Geometry check sheet. Reference: the model listing, model coordinates, mm. Coordinates: 2 decimals unless noted, no trailing zeros. Write each loop counter-clockwise with the first axis right and the second up, starting at its lowest first coordinate (ties: lowest second). Pieces come first, ordered by that corner, then holes. Notation, with made-up numbers: (-18.5, 43.25) -> (-9.5, 43.25) arc R29 ccw to (-9.5, 77.25) -> close; hole circle Ø11 at (41, -29). An arc over 180 degrees is marked (long way). Answer as CSV lines item,"result".
```python
from build123d import *

# Parameters (mm, degrees)
F1_DEPTH = 3
F2_DEPTH = 25
F3_R     = 7
F4_R     = 100
F5_R     = 7
F6_R     = 3


# Not quite as in the source:
# - a feature names something its author has since deleted; it is built from what else it names


with BuildPart() as f1:
    # F0 (on Front) → F1 (new body)
    with BuildSketch(Plane.XZ):
        with BuildLine():
            Line((-28.5062876117, 71.7030383349), (-23.3711215756, 71.5975238881))
            ThreePointArc((-23.3711215756, 71.5975238881), (-24.6315082315, 75.5227380174), (-26.6928125912, 79.0930187933))
            ThreePointArc((-26.6928125912, 79.0930187933), (-46.4685424733, 86.625019162), (-61.3664115867, 71.5962461648))
            Line((-61.3664115867, 71.5962461648), (-56.3664115867, 71.5913571682))
            ThreePointArc((-56.3664115867, 71.5913571682), (-42.4756351566, 81.447422187), (-28.5062876117, 71.7030383349))
        make_face()
        with BuildLine():
            ThreePointArc((-61.3664115867, 71.5962461648), (-42.3681277411, 52.5998806027), (-23.3711215756, 71.5975238881))
            Line((-23.3711215756, 71.5975238881), (-28.5062876117, 71.7030383349))
            ThreePointArc((-28.5062876117, 71.7030383349), (-35.0280474509, 67.9936357913), (-42.4162418185, 66.6868830915))
            ThreePointArc((-42.4162418185, 66.6868830915), (-49.8149115034, 67.9342855664), (-56.3664115867, 71.5913571682))
            Line((-56.3664115867, 71.5913571682), (-61.3664115867, 71.5962461648))
        make_face()
        with BuildLine():
            ThreePointArc((-42.4162418185, 66.6868830915), (-35.0280474509, 67.9936357913), (-28.5062876117, 71.7030383349))
            ThreePointArc((-28.5062876117, 71.7030383349), (-42.4756351566, 81.447422187), (-56.3664115867, 71.5913571682))
            ThreePointArc((-56.3664115867, 71.5913571682), (-49.8149115034, 67.9342855664), (-42.4162418185, 66.6868830915))
        make_face()
        with BuildLine():
            Line((-20.8711215756, 71.5975236603), (-23.3711215756, 71.5975238881))
            ThreePointArc((-23.3711215756, 71.5975238881), (-42.3681277411, 52.5998806027), (-61.3664115867, 71.5962461648))
            Line((-61.3664115867, 71.5962461648), (-63.866411581, 71.5960777947))
            ThreePointArc((-63.866411581, 71.5960777947), (-63.6941147241, 68.8812286525), (-63.1803487139, 66.2098738354))
            ThreePointArc((-63.1803487139, 66.2098738354), (-48.9397473345, 51.1287456375), (-28.5819229469, 55.1029300277))
            ThreePointArc((-28.5819229469, 55.1029300277), (-22.8939959961, 62.4935676044), (-20.8711215756, 71.5975236602))
        make_face()
        with BuildLine():
            ThreePointArc((-26.6928125912, 79.0930187933), (-24.6315082315, 75.5227380174), (-23.3711215756, 71.5975238881))
            Line((-23.3711215756, 71.5975238881), (-20.8711215756, 71.5975236603))
            ThreePointArc((-20.8711215756, 71.5975236602), (-22.8939959961, 62.4935676044), (-28.5819229469, 55.1029300277))
            ThreePointArc((-28.5819229469, 55.1029300277), (-33.5715090435, 45.0303149316), (-38.6320985636, 34.9931849634))
            ThreePointArc((-38.6320985636, 34.9931849634), (-28.2353261857, 40.6242290748), (-18.8527258187, 47.819251244))
            ThreePointArc((-18.8527258187, 47.819251244), (-11.5073907557, 58.7139707043), (-8.9261215756, 71.5975225718))
            Line((-8.9261215756, 71.5975225718), (-11.6744206899, 71.5975225718))
            Line((-11.6744206899, 71.5975225718), (-11.6744206899, 74.0203762137))
            ThreePointArc((-11.6744206899, 74.0203762137), (-14.431706638, 81.8781100982), (-19.1607128583, 88.7325325952))
            ThreePointArc((-19.1607128583, 88.7325325952), (-48.5320541227, 98.3962580044), (-71.9061774941, 78.1548738354))
            Line((-71.9061774941, 78.1548738354), (-107.2845857728, 78.1548738354))
            Line((-107.2845857728, 78.1548738354), (-119.2295857724, 78.1548738354))
            Line((-119.2295857724, 78.1548738354), (-119.2295857724, 66.2098738355))
            Line((-119.2295857724, 66.2098738355), (-119.2295857724, 47.819251244))
            ThreePointArc((-119.2295857724, 47.819251244), (-113.3445755267, 44.456364285), (-107.2845857724, 41.4201036786))
            Line((-107.2845857724, 41.4201036786), (-107.2845857724, 66.2098738354))
            Line((-107.2845857724, 66.2098738354), (-68.5864427672, 66.2098738354))
            Line((-68.5864427672, 66.2098738354), (-63.1803487138, 66.2098738354))
            ThreePointArc((-63.1803487139, 66.2098738354), (-63.6941147241, 68.8812286525), (-63.866411581, 71.5960777947))
            Line((-63.866411581, 71.5960777947), (-61.3664115867, 71.5962461648))
            ThreePointArc((-61.3664115867, 71.5962461648), (-46.4685424733, 86.625019162), (-26.6928125912, 79.0930187933))
        make_face()
        with BuildLine():
            Line((-11.6744206899, 71.5975225718), (-8.9261215756, 71.5975225718))
            ThreePointArc((-8.9261215756, 71.5975225718), (-13.1797411051, 80.6808937542), (-19.1607128583, 88.7325325952))
            ThreePointArc((-19.1607128583, 88.7325325952), (-14.431706638, 81.8781100982), (-11.6744206899, 74.0203762137))
            Line((-11.6744206899, 74.0203762137), (-11.6744206899, 71.5975225718))
        make_face()
        with BuildLine():
            Line((-119.2295857724, 47.819251244), (-119.2295857724, 37.819251244))
            Line((-119.2295857724, 37.819251244), (-97.7339796794, 37.4339680289))
            ThreePointArc((-97.7339796794, 37.4339680289), (-102.5508909325, 39.3273444167), (-107.2845857724, 41.4201036786))
            ThreePointArc((-107.2845857724, 41.4201036786), (-113.3445755267, 44.456364285), (-119.2295857724, 47.819251244))
        make_face()
        with BuildLine():
            ThreePointArc((-38.6320985636, 34.9931849634), (-33.5715090435, 45.0303149316), (-28.5819229469, 55.1029300277))
            ThreePointArc((-28.5819229469, 55.1029300277), (-48.9397473345, 51.1287456375), (-63.1803487139, 66.2098738354))
            Line((-63.1803487138, 66.2098738354), (-68.5864427672, 66.2098738354))
            Line((-68.5864427672, 66.2098738354), (-107.2845857724, 66.2098738354))
            Line((-107.2845857724, 66.2098738354), (-107.2845857724, 41.4201036786))
            ThreePointArc((-107.2845857724, 41.4201036786), (-102.5508909325, 39.3273444167), (-97.7339796794, 37.4339680289))
            Line((-97.7339796794, 37.4339680289), (-71.3664115866, 36.9613606799))
            Line((-71.3664115866, 36.9613606799), (-71.3664115866, 30.923581687))
            ThreePointArc((-71.3664115866, 30.923581687), (-54.830296618, 31.5993469164), (-38.6320985636, 34.9931849634))
        make_face()
    extrude(amount=F1_DEPTH)

    # F0 (on Front) → F2 (cut)
    with BuildSketch(Plane.XZ):
        with BuildLine():
            ThreePointArc((-42.4162418185, 66.6868830915), (-35.0280474509, 67.9936357913), (-28.5062876117, 71.7030383349))
            ThreePointArc((-28.5062876117, 71.7030383349), (-42.4756351566, 81.447422187), (-56.3664115867, 71.5913571682))
            ThreePointArc((-56.3664115867, 71.5913571682), (-49.8149115034, 67.9342855664), (-42.4162418185, 66.6868830915))
        make_face()
    extrude(amount=F2_DEPTH, mode=Mode.SUBTRACT)

    # F3
    f3_edges = [f1.edges().sort_by_distance(p)[0] for p in [
        (-8.926122, -1.5, 71.597523),
        (-119.229586, -1.5, 37.819251),
    ]]
    fillet(f3_edges, radius=F3_R)

    # F4
    f4_edges = [f1.edges().sort_by_distance(p)[0] for p in [
        (-71.906177, -1.5, 78.154874),
    ]]
    fillet(f4_edges, radius=F4_R)

    # F5
    f5_edges = [f1.edges().sort_by_distance(p)[0] for p in [
        (-119.229586, -1.5, 78.154874),
    ]]
    fillet(f5_edges, radius=F5_R)

    # F6
    f6_edges = [f1.edges().sort_by_distance(p)[0] for p in [
        (-71.366412, -1.5, 36.961361),
        (-71.366412, -1.5, 30.923582),
    ]]
    fillet(f6_edges, radius=F6_R)


solid = f1.part
```
Item 1: Cross-section at A-A, the plane x = -51. Record the cut outline in (y, z), plus the area to 3 significant figures.
Responses:
outline,"(-3, 32.15) -> (0, 32.15) -> (0, 68.39) -> (-3, 68.39) -> close; (-3, 78.7) -> (0, 78.7) -> (0, 97.8) -> (-3, 97.8) -> close"
area,"166 mm2"
Item 2: Release check for a two-part mould opening along X. For faces 1 (the flat face through (-65, -3, 65)), 2 (the cylindrical face through (-70.524, -1.521, 31.758)), 3 (the cylindrical face through (-42.222, -1.479, 81.446)) record: +X half, -X half, draft (parallel to the pull), parting line (faces both ways), or undercut.
Responses:
face 1,"draft"
face 2,"-X half"
face 3,"undercut"
Item 3: Cross-section at B-B, the plane z = 69. Record the cut outline in (x, y), plus the area to 3 significant figures.
Responses:
outline,"(-119.23, -3) -> (-52.33, -3) -> (-52.33, 0) -> (-119.23, 0) -> close; (-32.68, -3) -> (-9.03, -3) -> (-9.03, 0) -> (-32.68, 0) -> close"
area,"272 mm2"
Item 4: Cross-section at D-D, the plane x = -24.5. Record the cut outline in (y, z), plus the area to 3 significant figures.
Responses:
outline,"(-3, 43.21) -> (0, 43.21) -> (0, 93.42) -> (-3, 93.42) -> close"
area,"151 mm2"
Item 5: Cross-section at C-C, the plane z = 52.5. Record the cut outline in (x, y), plus the area to 3 significant figures.
Responses:
outline,"(-119.23, -3) -> (-14.92, -3) -> (-14.92, 0) -> (-119.23, 0) -> close"
area,"313 mm2"
Item 6: Depth check by flat-ended pin: pin 1 Ø1 at (x, y) = (-43.5, -1) entering from -Z. Enter the tip coordinate at first touch or a pass-through.
Responses:
pin 1,"stops at z = 33.56"
Item 7: Thickness scan on probe 1 along X at (y, z) = (-2.25, 69); probe 2 along Z at (x, y) = (-30.5, -2.1); probe 3 along Z at (x, y) = (-46, -0.35). Record the ranges inside material, lowest first.
Responses:
probe 1,"x = -119.23 to -52.33, -32.68 to -9.03"
probe 2,"z = 39.21 to 70.24, 75.43 to 96.67"
probe 3,"z = 33.1 to 66.97, 81.01 to 98.8"
